For this review, take the finished solid that the model builds, in its own axes (mm). Give positions to 0.01 mm unless a question says otherwise; leave off trailing zeros. Use a Markdown table: item, result. Add a question column.
1) Wall thickness on L1, parallel to Z at x = 66, y = 189; L2, parallel to Z at x = 86, y = 110.5; L3, parallel to X at y = 70.5, z = 2.5: over which ranges is each line inside the solid? List them lowest first.
2) Clearance check with flat-ended pins moving along their axes: P1, Ø1.5, axis at y = 173.5, z = -2.5, coming from the -X side; P2, Ø6.5, axis at x = 148, z = 0.5, coming from the -Y side; P3, Ø4, axis at y = 168, z = 1.5, coming from the -X side; P4, Ø4, axis at y = 207, z = -5.5, coming from the +X side. State where each tip first meets the part, or that it passes through.
3) Mouldability with a two-part tool opening along Y and no side actions: class faces 1 (the face through (108, 250, 0)), 2 (the face through (57, 0, 0)), 3 (the face through (149, 225, 0)) as released by +Y, released by -Y, zero draft, split by the parting line, or undercut.
```python
from build123d import *

# Parameters (mm, degrees)
CUT_EXTRUDE1_DEPTH      = 303.533691694
CUT_EXTRUDE1_DEPTH_BACK = 303.533691694


with BuildPart() as part:
    # Sketch2 → Loft1 section 0
    with BuildSketch(Plane(origin=(0, 0, 0), x_dir=(1, 0, 0), z_dir=(0, 1, 0))):
        with BuildLine():
            add(Edge.make_bspline(
                [(0, 0), (0.357433553, 1.567842951), (1.917970176, 4.160229764), (5.97481653, 6.081249697), (9.685317154, 7.498428782), (13.560078119, 8.488450032), (17.359013279, 9.274437737), (21.537080113, 9.926762724), (26.46178465, 10.495714484), (33.030088427, 11.004191676), (39.777903449, 11.237535202), (48.881830343, 11.276440135), (58.76193613, 11.001555412), (68.683481214, 10.411026067), (82.689863985, 9.343738865), (94.136580366, 8.168132094), (108.892414504, 6.408281033), (116.550975745, 5.416254952), (123.975633155, 4.354289335), (127.960081342, 3.77052037), (132.393799107, 3.105793902), (137.115401047, 2.40243394), (143.03529364, 1.468316053), (147.203728737, 0.596703087), (150, 0)],
                knots=[0, 0, 0, 0, 0.031271315, 0.055076604, 0.085653186, 0.108857761, 0.132714605, 0.161157924, 0.191102095, 0.229169149, 0.289322728, 0.322456152, 0.406317058, 0.481621487, 0.515848821, 0.679661265, 0.705502791, 0.805025067, 0.829931294, 0.851453308, 0.883388416, 0.917173131, 0.944349664, 1, 1, 1, 1], degree=3))
            add(Edge.make_bspline(
                [(0, 0), (0.394064241, -1.54877785), (1.863432045, -4.108329327), (5.28724909, -5.736171), (8.233222924, -6.999318685), (11.439608234, -7.961073986), (14.837636919, -8.774678376), (18.226738528, -9.412867336), (21.607899865, -9.923992079), (25.17739935, -10.35155024), (30.263863608, -10.813990829), (36.567415813, -11.154786303), (45.633644275, -11.313399436), (54.659951216, -11.138633145), (65.729134774, -10.617890693), (80.628353886, -9.553465623), (94.39151788, -8.136116187), (108.235367187, -6.487796867), (115.481434177, -5.556138542), (124.038094924, -4.350742236), (129.185840061, -3.589034499), (134.229817914, -2.830310801), (137.671437841, -2.315360587), (140.909856219, -1.801519139), (145.017744862, -1.058252808), (147.972088501, -0.42879218), (150, 0)],
                knots=[0, 0, 0, 0, 0.031458743, 0.053377779, 0.072332266, 0.094059262, 0.118322991, 0.140338064, 0.161137525, 0.18485863, 0.210283619, 0.260514048, 0.30767032, 0.386712656, 0.436156502, 0.523300177, 0.677353161, 0.705359806, 0.794596405, 0.819513727, 0.8735115, 0.895859044, 0.9187711, 0.941229566, 0.959662244, 1, 1, 1, 1], degree=3))
        make_face()
    # Sketch3 → Loft1 section 1
    with BuildSketch(Plane(origin=(0, 250, 0), x_dir=(1, 0, 0), z_dir=(0, 1, 0))):
        with BuildLine():
            add(Edge.make_bspline(
                [(70, 0), (69.998695985, 0.55955733), (70.442205932, 1.260933045), (71.2121543, 1.885639789), (72.176569209, 2.500244125), (73.360859293, 3.018557927), (75.122720532, 3.618750694), (76.659068738, 4.023634354), (78.453879641, 4.413670772), (80.755673074, 4.834011856), (83.864457382, 5.25286849), (87.961435036, 5.633828774), (93.124785839, 5.92406083), (99.760074537, 6.045439608), (107.468637421, 5.921147675), (115.967916909, 5.556531892), (125.064057366, 4.966684256), (134.169678192, 4.212287311), (143.356076333, 3.327498387), (150.536726311, 2.550254072), (156.205971927, 1.886416966), (159.803934974, 1.44813753), (164.387726212, 0.858989173), (167.770673402, 0.429320596), (170, 0)],
                knots=[0, 0, 0, 0, 0.015533955, 0.02314791, 0.028948177, 0.048950772, 0.060740409, 0.083424122, 0.095372754, 0.114483795, 0.151867659, 0.187126741, 0.23485952, 0.303156584, 0.381272081, 0.460411987, 0.552057215, 0.647968854, 0.727745971, 0.822090373, 0.859296949, 0.894761026, 0.928143313, 0.994524953, 0.994524953, 0.994524953, 0.994524953], degree=3))
            add(Edge.make_bspline(
                [(70, 0), (69.998695985, -0.55955733), (70.442205932, -1.260933045), (71.2121543, -1.885639789), (72.176569209, -2.500244125), (73.360859293, -3.018557927), (75.122720532, -3.618750694), (76.659068738, -4.023634354), (78.453879641, -4.413670772), (80.755673074, -4.834011856), (83.864457382, -5.25286849), (87.961435036, -5.633828774), (93.124785839, -5.92406083), (99.760074537, -6.045439608), (107.468637421, -5.921147675), (115.967916909, -5.556531892), (125.064057366, -4.966684256), (134.169678192, -4.212287311), (143.356076333, -3.327498387), (150.536726311, -2.550254072), (156.205971927, -1.886416966), (159.803934974, -1.44813753), (164.387726212, -0.858989173), (167.770673402, -0.429320596), (170, 0)],
                knots=[0, 0, 0, 0, 0.015533955, 0.02314791, 0.028948177, 0.048950772, 0.060740409, 0.083424122, 0.095372754, 0.114483795, 0.151867659, 0.187126741, 0.23485952, 0.303156584, 0.381272081, 0.460411987, 0.552057215, 0.647968854, 0.727745971, 0.822090373, 0.859296949, 0.894761026, 0.928143313, 0.994524953, 0.994524953, 0.994524953, 0.994524953], degree=3))
        make_face()
    loft()

    # Sketch4 → Cut-Extrude1 (cut, two sides: drawn at the far end of the back side and taken through both)
    with BuildSketch(Plane.XY.offset(-CUT_EXTRUDE1_DEPTH_BACK)):
        Polygon((152, 25), (108.5, 25), (136.5, 225), (168, 225), align=None)
    extrude(amount=CUT_EXTRUDE1_DEPTH + CUT_EXTRUDE1_DEPTH_BACK, mode=Mode.SUBTRACT)


solid = part.part
```
Checked values:
| question | item | result |
|---|---|---|
| 1 | L1 | -5.99 to 5.99 |
| 1 | L2 | -8.45 to 8.45 |
| 1 | L3 | 20.96 to 114.87 |
| 2 | P1 | x = 49.36 |
| 2 | P2 | y = 0 |
| 2 | P3 | x = 46.64 |
| 2 | P4 | x = 134.19 |
| 3 | face 1 | released by +Y |
| 3 | face 2 | released by -Y |
| 3 | face 3 | undercut |
